Check sheet for the modelled part. Datum: model origin and axes. Units: mm. A direction names the side the tool comes from. Round coordinates to 2 decimals unless told otherwise and drop trailing zeros. Loops run counter-clockwise (first coordinate to the right, second up) from the corner with the lowest first, then second, coordinate; pieces in that order, holes last. Notation, with made-up numbers: (-18, -31.75) - (39, -31.75) arc R17 ccw to (39, -20.75) - close; hole circle Ø4 at (-26.5, -23). An arc over 180 degrees is marked (long way). Put each result on its own line as item: value. Start each with the question number.
Item 1: Section check A-A, the plane x = -58. Record the cut outline in (y, z).
Item 2: Gauge pin test, flat ends, axial feed: pin 1 Ø10.5 at (x, y) = (-68, 277) entering from +Z; pin 2 Ø10.5 at (x, y) = (-64.5, 282.5) entering from -Z; pin 3 Ø8 at (x, z) = (-27.5, 3.5) entering from +Y. Record the tip position at first contact, or that the pin passes through.
Item 3: Material ranges on line 1 along Y through (x, z) = (-38, 23.5); line 2 along Z through (x, y) = (-56.5, 273), recorded low to high.
Item 4: Section check D-D, the plane x = -24. Record the cut outline in (y, z).
Item 5: Section check C-C, the plane z = -6. Record the cut outline in (x, y), and give its area (3 significant figures).
Item 6: Draft check along X on faces 1 (the flat face through (-1, 0, 0)), 2 (the flat face through (-45.1, 281.35, -9.86)), 3 (the flat face through (-89, 134, 0)). Enter one of: pulls with the +X half, pulls with the -X half, needs draft (parallel to the pull), parting line crosses it, or undercut.
Item 7: Tool access check on faces 4 (the flat face through (63, 281, -20)), 5 (the flat face through (79.74, 281.35, 10.14)), 6 (the flat face through (-79.9, 281.35, 9.86)), 7 (the flat face through (-1, 271, 0)), 8 (the flat face through (-45.26, 281.35, 10.14)). Record the directions out of +Z, -Z, +X, -X, +Y, -Y that give a thin tool (end or side, any length) a straight path to the whole face; none if there is none.
Item 8: Section check B-B, the plane z = 15. Record the cut outline in (x, y), and give its area (3 significant figures).
from build123d import *

# Parameters (mm, degrees)
SKETCH1_W           = 178
SKETCH1_H           = 71
BOSS_EXTRUDE1_DEPTH = 271
BOSS_EXTRUDE2_DEPTH = 21


with BuildPart() as part:
    # Sketch1 → Boss-Extrude1 (new body)
    with BuildSketch(Plane(origin=(0, 0, 0), x_dir=(1, 0, 0), z_dir=(0, 1, 0))):
        Rectangle(SKETCH1_W, SKETCH1_H)
    extrude(amount=BOSS_EXTRUDE1_DEPTH)

    # Sketch2 → Boss-Extrude2 (add)
    with BuildSketch(Plane(origin=(0, 271, 0), x_dir=(1, 0, 0), z_dir=(0, 1, 0))):
        Polygon((-39.405989232, 0), (-50.952994616, 20), (-74.047005384, 20), (-85.594010768, 0), (-74.047005384, -20), (-50.952994616, -20), align=None)
        Polygon((85.594010768, 0), (74.047005384, 20), (50.952994616, 20), (39.405989232, 0), (50.952994616, -20), (74.047005384, -20), align=None)
    extrude(amount=BOSS_EXTRUDE2_DEPTH)


solid = part.part
Check result:
1. outline: (0, -35.5) - (271, -35.5) - (271, -20) - (292, -20) - (292, 20) - (271, 20) - (271, 35.5) - (0, 35.5) - close
2. pin 1: z = 20
2. pin 2: z = -20
2. pin 3: y = 271
3. line 1: 0 to 271
3. line 2: -20 to 20
4. outline: (0, -35.5) - (271, -35.5) - (271, 35.5) - (0, 35.5) - close
5. outline: (-89, 0) - (89, 0) - (89, 271) - (82.13, 271) - (82.13, 292) - (42.87, 292) - (42.87, 271) - (-42.87, 271) - (-42.87, 292) - (-82.13, 292) - (-82.13, 271) - (-89, 271) - close
5. area: 49,900 mm²
6. face 1: needs draft
6. face 2: undercut
6. face 3: pulls with the -X half
7. face 4: -Z, +X, -X, +Y
7. face 5: +Z, +X, +Y
7. face 6: +Z, -X, +Y
7. face 7: +Y
7. face 8: +Z, +Y
8. outline: (-89, 0) - (89, 0) - (89, 271) - (76.93, 271) - (76.93, 292) - (48.07, 292) - (48.07, 271) - (-48.07, 271) - (-48.07, 292) - (-76.93, 292) - (-76.93, 271) - (-89, 271) - close
8. area: 49,500 mm²
